Read the model definition and answer for the solid it produces. Units are mm, in the model's axes. Round coordinates to 2 decimals unless told otherwise and drop trailing zeros. Answer as CSV lines item,"result".
```python
from build123d import *

# Parameters (mm, degrees)
SKETCH1_W                  = 95
SKETCH1_H                  = 8.75
BOSS_EXTRUDE1_DEPTH        = 10
F_2_8_2_8_DIAMETER_HOLE1_D = 2.8
F_1_4_1_4_DIAMETER_HOLE1_D = 1.4
LPATTERN1_COUNT            = 32
LPATTERN1_PITCH            = 2.54


with BuildPart() as part:
    # Sketch1 → Boss-Extrude1 (new body)
    with BuildSketch(Plane(origin=(0, 0, 0), x_dir=(1, 0, 0), z_dir=(0, 1, 0))):
        Rectangle(SKETCH1_W, SKETCH1_H)
    extrude(amount=BOSS_EXTRUDE1_DEPTH)

    # Ø2.8 (2.8) Diameter Hole1 (through all)
    with Locations(Plane(origin=(-45, 10, -0.3), x_dir=(0, 0, 1), z_dir=(0, 1, 0))):
        with Locations((0, 0), (0, 90)):
            Hole(F_2_8_2_8_DIAMETER_HOLE1_D / 2)

    # Ø1.4 (1.4) Diameter Hole1 (through all)
    with Locations(Plane(origin=(-39.37, 10, -2.54), x_dir=(0, 0, 1), z_dir=(0, 1, 0))):
        with Locations((0, 0), (2.54, 0), (5.08, 0)):
            f_1_4_1_4_diameter_hole1 = Hole(F_1_4_1_4_DIAMETER_HOLE1_D / 2)

    # LPattern1: Ø1.4 (1.4) Diameter Hole1 ×32
    with Locations(*[(i * LPATTERN1_PITCH, 0, 0) for i in range(1, LPATTERN1_COUNT)]):
        add(f_1_4_1_4_diameter_hole1, mode=Mode.SUBTRACT)


solid = part.part
```
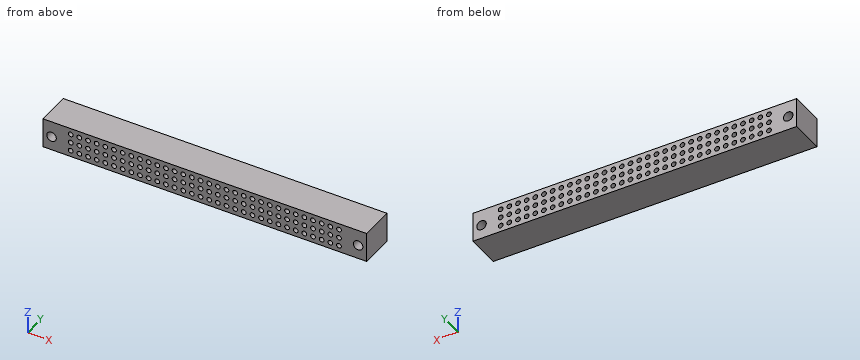
Item 1: A flat-ended cylindrical pin translates along its axis: pin 1 (1.1 mm diameter, centred on x = -29.21, z = 2.54, fed in from -Y). Find the tip coordinate at first contact, or state that the pin passes through.
Ans:
pin 1,"through"
Item 2: A cutting plane is placed at A-A, the plane y = 6. Give the number of separate pieces and of enclosed holes in the cut face, and give its area (3 significant figures).
Ans:
separate pieces,"1"
enclosed holes,"98"
area,"671 mm2"
Item 3: Find the intervals of material crossed by probe 1 along Z at (x, y) = (34.29, 4) (3 decimals); probe 2 along Z at (x, y) = (24, 6.75) (3 decimals), in increasing order. Write a range as [from, to].
Ans:
probe 1,"[-4.375, -3.24], [-1.84, -0.7], [0.7, 1.84], [3.24, 4.375]"
probe 2,"[-4.375, -3.228], [-1.852, -0.688], [0.688, 1.852], [3.228, 4.375]"
